Could you check a few things on this model? Use its own coordinates, in mm. A direction names the side the tool comes from. Coordinates: 2 decimals unless noted, no trailing zeros. Loops run counter-clockwise (first coordinate to the right, second up) from the corner with the lowest first, then second, coordinate; pieces in that order, holes last. Notation, with made-up numbers: (76, -20.5) -> (126, -20.5) arc R8 ccw to (126, -10.5) -> close; hole circle Ø9 at (21, 4). An arc over 180 degrees is marked (long way). One line per question, with ' | ' between items.
from build123d import *

# Parameters (mm, degrees)
SKETCH_1_W      = 75.1
SKETCH_1_H      = 150.3
EXTRUDE_1_DEPTH = 11
FILLET_1_R      = 12
FILLET_2_R      = 1.8
EXTRUDE_2_DEPTH = 2.5


with BuildPart() as part:
    # 草图1 → 凸台-拉伸1 (new body)
    with BuildSketch(Plane(origin=(0, 0, 0), x_dir=(1, 0, 0), z_dir=(0, 1, 0))):
        Rectangle(SKETCH_1_W, SKETCH_1_H)
    extrude(amount=EXTRUDE_1_DEPTH)

    # 圆角1
    fillet_1_edges = [part.edges().sort_by_distance(p)[0] for p in [
        (37.55, 5.5, 75.15),
        (-37.55, 5.5, 75.15),
        (-37.55, 5.5, -75.15),
        (37.55, 5.5, -75.15),
    ]]
    fillet(fillet_1_edges, radius=FILLET_1_R)

    # 圆角2
    fillet_2_edges = [part.edges().sort_by_distance(p)[0] for p in [
        (0, 0, -75.15),
        (37.55, 0, 0),
        (0, 0, 75.15),
        (-37.55, 0, 0),
        (-34.035281374, 0, -71.635281374),
        (-34.035281374, 0, 71.635281374),
        (34.035281374, 0, 71.635281374),
        (34.035281374, 0, -71.635281374),
    ]]
    fillet(fillet_2_edges, radius=FILLET_2_R)

    # 草图2 → 凸台-拉伸2 (add)
    with BuildSketch(Plane.XZ):
        with BuildLine():
            Line((21.45, -29.85), (5.45, -29.85))
            ThreePointArc((5.45, -29.85), (-3.035281374, -33.364718626), (-6.55, -41.85))
            Line((-6.55, -41.85), (-6.55, -58.65))
            ThreePointArc((-6.55, -58.65), (-3.035281374, -67.135281374), (5.45, -70.65))
            Line((5.45, -70.65), (21.45, -70.65))
            ThreePointArc((21.45, -70.65), (29.935281374, -67.135281374), (33.45, -58.65))
            Line((33.45, -58.65), (33.45, -41.85))
            ThreePointArc((33.45, -41.85), (29.935281374, -33.364718626), (21.45, -29.85))
        make_face()
    extrude(amount=EXTRUDE_2_DEPTH)


solid = part.part
1) If we section it at A-A on x = 18: Please give me the cut outline in (y, z), and give its area (3 significant figures).
Data:
outline: (-2.5, -70.65) -> (0, -70.65) -> (0, -73.35) arc R1.8 ccw to (1.8, -75.15) -> (11, -75.15) -> (11, 75.15) -> (1.8, 75.15) arc R1.8 ccw to (0, 73.35) -> (0, -29.85) -> (-2.5, -29.85) -> close | area: 1,750 mm²
2) If we section it at C-C on x = -23.5: Please give me the cut outline in (y, z).
Data:
outline: (0, -73.35) arc R1.8 ccw to (1.8, -75.15) -> (11, -75.15) -> (11, 75.15) -> (1.8, 75.15) arc R1.8 ccw to (0, 73.35) -> close
3) On a 3-axis mill with a long thin cutter (end or side, diameter ignored), from which of +Z, -Z, +X, -X, +Y, -Y can I reach the whole of each face in a straight line? I mean faces 1 (the face through (-3.13, -1.23, -67.04)), 2 (the face through (29.84, -1.23, -67.23)), 3 (the face through (-2.94, -1.23, -33.27)). Say none if no direction works.
Data:
face 1: -Z, -X, -Y | face 2: -Z, +X, -Y | face 3: +Z, -X, -Y
4) If we section it at B-B on z = -22.5: Please give me the cut outline in (x, y).
Data:
outline: (-37.55, 1.8) arc R1.8 ccw to (-35.75, 0) -> (35.75, 0) arc R1.8 ccw to (37.55, 1.8) -> (37.55, 11) -> (-37.55, 11) -> close
5) I'm going to push flat-ended pins straight in: pin 1 Ø0.8 at (x, y) = (12.5, -0.5) entering from -Z; pin 2 Ø1.5 at (x, y) = (29, 2) entering from -Z; pin 3 Ø2 at (x, y) = (13, -1.5) entering from +Z. Where does each tip first touch, or does it pass through?
Data:
pin 1: z = -70.65 | pin 2: z = -74.84 | pin 3: z = -29.85
6) I need wall thicknesses on line 1 along Y through (x, z) = (-26.5, -32.5); line 2 along X through (y, z) = (1.5, -44); line 3 along Z through (x, y) = (-4.5, 0.75). Which ranges of each line are inside material? Lowest first, please. Write a range as from..to.
Data:
line 1: 0..11 | line 2: -37.52..37.52 | line 3: -74.81..74.81
7) If we section it at D-D on x = 1: Please give me the cut outline in (y, z), and give its area (3 significant figures).
Data:
outline: (-2.5, -69.79) -> (0, -69.79) -> (0, -73.35) arc R1.8 ccw to (1.8, -75.15) -> (11, -75.15) -> (11, 75.15) -> (1.8, 75.15) arc R1.8 ccw to (0, 73.35) -> (0, -30.71) -> (-2.5, -30.71) -> close | area: 1,750 mm²
